from build123d import *

# Parameters (mm, degrees)
F1_DEPTH  = 1181.1
F2_W      = 228.6
F2_H      = 482.6
F3_DEPTH  = 25.4
F4_SIZE   = 50.8
F5_W      = 254
F5_H      = 482.6
F5_R      = 17.526
F6_DEPTH  = 31.75
F7_W      = 114.3
F7_H      = 25.4
F8_DEPTH  = 203.2
F10_DEPTH = 381.001
F13_W     = 25.4
F13_H     = 228.6
F14_DEPTH = 269.875
F15_R     = 14.2875
F15_R_2   = 36.5125
F15_W     = 25.4
F15_H     = 228.6
F16_DEPTH = 50.8
F17_W     = 361.3794893026
F17_H     = 323.3922393799
F18_DEPTH = 6.35
F20_R     = 30.1625
F21_DEPTH = 50.8
F23_DEPTH = 6.35


with BuildPart() as f1:
    # F0 (on Right) → F1 (new body, symmetric)
    with BuildSketch(Plane.YZ):
        with BuildLine():
            Line((76.2, 152.4), (-76.2, 152.4))
            ThreePointArc((-76.2, 152.4), (-94.1605122421, 144.9605122421), (-101.6, 127))
            Line((-101.6, 127), (-101.6, -127))
            ThreePointArc((-101.6, -127), (-94.1605122421, -144.9605122421), (-76.2, -152.4))
            Line((-76.2, -152.4), (76.2, -152.4))
            ThreePointArc((76.2, -152.4), (94.1605122421, -144.9605122421), (101.6, -127))
            Line((101.6, -127), (101.6, 127))
            ThreePointArc((101.6, 127), (94.1605122421, 144.9605122421), (76.2, 152.4))
        make_face()
        with BuildLine():
            ThreePointArc((-88.9, 127), (-85.1802561211, 135.9802561211), (-76.2, 139.7))
            Line((-76.2, 139.7), (76.2, 139.7))
            ThreePointArc((76.2, 139.7), (85.1802561211, 135.9802561211), (88.9, 127))
            Line((88.9, 127), (88.9, -127))
            ThreePointArc((88.9, -127), (85.1802561211, -135.9802561211), (76.2, -139.7))
            Line((76.2, -139.7), (-76.2, -139.7))
            ThreePointArc((-76.2, -139.7), (-85.1802561211, -135.9802561211), (-88.9, -127))
            Line((-88.9, -127), (-88.9, 127))
        make_face(mode=Mode.SUBTRACT)
    extrude(amount=F1_DEPTH, both=True)

    # F2 (on face) → F3 (join)
    with BuildSketch(Plane.YZ.offset(1181.1)):
        with Locations((-12.7, 0)):
            Rectangle(F2_W, F2_H)
    extrude(amount=F3_DEPTH)

    # F4
    f4_edges = [f1.edges().sort_by_distance(p)[0] for p in [
        (1193.8, -127, 241.3),
        (1193.8, -127, -241.3),
    ]]
    chamfer(f4_edges, length=F4_SIZE)

    # F5 (on face) → F6 (join)
    with BuildSketch(Plane(origin=(0, 101.6, 0), x_dir=(-1, 0, 0), z_dir=(0, 1, 0))):
        with Locations((-1193.8, 0)):
            Rectangle(F5_W, F5_H)
        with Locations((-1270, -203.2)):
            Circle(F5_R, mode=Mode.SUBTRACT)
        with Locations((-1117.6, -203.2)):
            Circle(F5_R, mode=Mode.SUBTRACT)
        with Locations((-1270, 50.8)):
            Circle(F5_R, mode=Mode.SUBTRACT)
        with Locations((-1270, 203.2)):
            Circle(F5_R, mode=Mode.SUBTRACT)
        with Locations((-1117.6, 203.2)):
            Circle(F5_R, mode=Mode.SUBTRACT)
    extrude(amount=F6_DEPTH)

    # F7 (on face) → F8 (join)
    with BuildSketch(Plane.XZ.offset(-101.6)):
        with Locations((1263.65, 127)):
            Rectangle(F7_W, F7_H)
        with Locations((1263.65, -127)):
            Rectangle(F7_W, F7_H)
    extrude(amount=F8_DEPTH)

    # F9 (on face) → F10 (cut, through all)
    with BuildSketch(Plane.XY.offset(139.7)):
        Polygon((1219.2, -101.6), (1320.8, -101.6), (1320.8, 101.6), align=None)
    extrude(amount=-F10_DEPTH, mode=Mode.SUBTRACT)


with BuildPart() as f11_1:
    # F11: instance of F1
    add(f1.part.mirror(Plane.YZ))


with BuildPart() as f1_1:
    add(f1.part)

    # F12: union F11_1
    add(f11_1.part)

    # F13 (on Right) → F14 (join, symmetric)
    with BuildSketch(Plane.YZ):
        with Locations((44.45, 266.7)):
            Rectangle(F13_W, F13_H)
    extrude(amount=F14_DEPTH, both=True)

    # F15 (on face) → F16 (join)
    with BuildSketch(Plane.YZ.offset(269.875)):
        with BuildLine():
            Line((57.15, 152.4), (101.6, 152.4))
            Line((101.6, 152.4), (101.6, 508))
            ThreePointArc((101.6, 508), (93.2355821831, 541.1443160075), (70.1455781359, 566.3506819121))
            Line((70.1455781359, 566.3506819121), (11.1025355163, 605.2018432352))
            ThreePointArc((11.1025355163, 605.2018432352), (-21.4155981852, 606.6267979039), (-38.1, 578.6788060024))
            Line((-38.1, 578.6788060024), (-101.6, 203.2))
            Line((-101.6, 203.2), (-101.6, 152.4))
            Line((-101.6, 152.4), (31.75, 152.4))
            Line((31.75, 152.4), (31.75, 381))
            Line((31.75, 381), (57.15, 381))
            Line((57.15, 381), (57.15, 152.4))
        make_face()
        with Locations((-6.35, 578.6788060024)):
            Circle(F15_R, mode=Mode.SUBTRACT)
        with Locations((31.75, 508)):
            Circle(F15_R_2, mode=Mode.SUBTRACT)
        with Locations((44.45, 266.7)):
            Rectangle(F15_W, F15_H)
    extrude(amount=F16_DEPTH)

    # F17 (on face) → F18 (cut)
    with BuildSketch(Plane.YZ.offset(320.675)):
        with Locations((24.2072567344, 587.1461196899)):
            Rectangle(F17_W, F17_H)
    extrude(amount=-F18_DEPTH, mode=Mode.SUBTRACT)


with BuildPart() as f19_1:
    # F19: instance of F1
    add(f1_1.part.mirror(Plane.YZ))


with BuildPart() as f1_2:
    add(f1_1.part)

    add(f19_1.part)  # F21 merges F19_1
    # F20 (on Right) → F21 (join, symmetric)
    with BuildSketch(Plane.YZ):
        with BuildLine():
            Line((-101.6, -215.9), (76.2, -215.9))
            Line((76.2, -215.9), (76.2, -152.4))
            Line((76.2, -152.4), (-101.6, -152.4))
            Line((-101.6, -152.4), (-101.6, -139.7))
            Line((-101.6, -139.7), (-101.6, -127))
            Line((-101.6, -127), (-101.6, -38.1))
            Line((-101.6, -38.1), (-320.5653923257, -25.4944669429))
            ThreePointArc((-320.5653923257, -25.4944669429), (-379.9951543899, -71.8802231262), (-341.724064813, -136.8329651646))
            Line((-341.724064813, -136.8329651646), (-101.6, -215.9))
        make_face()
        with Locations((-323.85, -82.55)):
            Circle(F20_R, mode=Mode.SUBTRACT)
    extrude(amount=F21_DEPTH, both=True)


with BuildPart() as f23:
    # F22 (on face) → F23 (new body)
    with BuildSketch(Plane.YZ.offset(50.8)):
        Polygon((-247.65, -212.9706889391), (-247.65, -82.55), (-247.65, 21.7781551182), (-439.1066730022, 21.7781551182), (-439.1066730022, -212.9706889391), align=None)
    extrude(amount=-F23_DEPTH)


with BuildPart() as f24_1:
    # F24: instance of F23
    add(f23.part.mirror(Plane.YZ))


with BuildPart() as f1_3:
    add(f1_2.part)

    # F25: cut F24_1, F23
    add(f24_1.part, mode=Mode.SUBTRACT)
    add(f23.part, mode=Mode.SUBTRACT)


solid = f1_3.part
Here's how the part is built. I have some questions about the finished solid (model axes, mm). A direction names the side the tool comes from. Give positions to 0.01 mm unless a question says otherwise; leave off trailing zeros. Order: outer loops, then holes, each group sorted by start corner. A loop starts at its lowest first (then second) coordinate and runs counter-clockwise, first axis right, second up. Notation, with made-up numbers: M -14,-10.5 L 4,-10.5 A14 ccw 4,10.5 Z; hole C -17,43 d9. An arc over 180 degrees is marked long. Answer as a JSON object with one key per item and string values. Group by question number.
1) Suppose I cut it at B-B, the plane y = -214.5. Write out the boundary of the cut face in (x, z).
2) We'd pull the mould along Z, two halves only. Please class faces 5 (the flat face through (1196, 133.35, 3)), 6 (the cylindrical face through (-291.789, 51.379, 538.787)), 7 (the flat face through (1264, 101.6, 2)), 8 (the cylindrical face through (291.79, -20.99, 606.85)): pulls with the +Z half, pulls with the -Z half, needs draft (parallel to the pull), parting line crosses it, or undercut.
3) On a 3-axis mill with a long thin cutter (end or side, diameter ignored), from which of +Z, -Z, +X, -X, +Y, -Y can I reach the whole of each face in a straight line? I mean faces 1 (the flat face through (1250, 24, -139.7)), 2 (the flat face through (50.8, -124, -142)), 3 (the flat face through (-1250, 24, -139.7)), 4 (the flat face through (1194, 82, 241.3)). Say none if no direction works.
4) Please list where these lines run through material, in increasing order: L1, parallel to X at y = 111, z = 50; L2, parallel to X at y = -113.5, z = -137.5; L3, parallel to X at y = 122, z = 203. Write a range as [from, to].
5) Suppose I cut it at A-A, the plane x = 393.5. Write out the boundary of the cut face in (y, z).
6) I'm going to push flat-ended pins straight in: pin 1 Ø2 at (x, y) = (-982, 67) entering from +Z; pin 2 Ø7.5 at (x, y) = (-285.5, -88.5) entering from -Z; pin 3 Ø14 at (x, z) = (-1212, 131.5) entering from -Y; pin 4 Ø6 at (x, y) = (56, -106.5) entering from +Z. Where does each tip first touch, or does it pass through?
Results found:
{
 "1": {"outline": "M -50.8,-178.72 L 50.8,-178.72 L 50.8,-31.6 L -50.8,-31.6 Z"},
 "2": {"face 5": "needs draft", "face 6": "undercut", "face 7": "undercut", "face 8": "pulls with the +Z half"},
 "3": {"face 1": "-Z, +X, -Y", "face 2": "-Z, -Y", "face 3": "-Z, -X, -Y", "face 4": "+Z, +X, +Y, -Y"},
 "4": {"L1": "[-1320.8, -1287.51], [-1252.49, -1066.8], [1066.8, 1252.49], [1287.51, 1320.8]", "L2": "[-1206.5, -1181.1], [-50.8, 50.8], [1181.1, 1206.5]", "L3": "[-1320.8, -1287.52], [-1252.48, -1135.12], [-1100.08, -1066.8], [1066.8, 1100.08], [1135.12, 1252.48], [1287.52, 1320.8]"},
 "5": {"outline": "M -101.6,-127 A25.4 ccw -76.2,-152.4 L 76.2,-152.4 A25.4 ccw 101.6,-127 L 101.6,127 A25.4 ccw 76.2,152.4 L -76.2,152.4 A25.4 ccw -101.6,127 Z; hole M -88.9,-127 A12.7 ccw -76.2,-139.7 L 76.2,-139.7 A12.7 ccw 88.9,-127 L 88.9,127 A12.7 ccw 76.2,139.7 L -76.2,139.7 A12.7 ccw -88.9,127 Z"},
 "6": {"pin 1": "z = 152.4", "pin 2": "z = -150.92", "pin 3": "y = -127", "pin 4": "through"}
}
